from build123d import *

# Parameters (mm, degrees)
F1_DEPTH = 12
F2_W     = 13
F2_H     = 5.9
F3_DEPTH = 6
F4_W     = 13
F4_H     = 2.9
F5_DEPTH = 2
F6_W     = 2
F6_H     = 2.9
F7_DEPTH = 2


with BuildPart() as f1:
    # F0 (on Top) → F1 (new body)
    with BuildSketch(Plane.XY):
        Polygon((0, 3), (0, 0), (45, 0), (45, -5), (0, -5), (0, -13), (50, -13), (50, 3), align=None)
    extrude(amount=F1_DEPTH)

    # F2 (on face) → F3 (cut)
    with BuildSketch(Plane.XZ.offset(13)):
        with Locations((8.5, 6)):
            Rectangle(F2_W, F2_H)
    extrude(amount=-F3_DEPTH, mode=Mode.SUBTRACT)

    # F4 (on face) → F5 (cut, through all)
    with BuildSketch(Plane.XZ.offset(7)):
        with Locations((8.5, 6)):
            Rectangle(F4_W, F4_H)
    extrude(amount=-F5_DEPTH, mode=Mode.SUBTRACT)

    # F6 (on face) → F7 (cut, through all)
    with BuildSketch(Plane(origin=(0, 0, 0), x_dir=(0, -1, 0), z_dir=(-1, 0, 0))):
        with Locations((6, 6)):
            Rectangle(F6_W, F6_H)
    extrude(amount=-F7_DEPTH, mode=Mode.SUBTRACT)


solid = f1.part
CAD build for the part. Positions are in the model's coordinates, mm. A direction names the side the tool comes from. Give positions to 0.01 mm unless a question says otherwise; leave off trailing zeros. Order: outer loops, then holes, each group sorted by start corner. A loop starts at its lowest first (then second) coordinate and runs counter-clockwise, first axis right, second up. Notation, with made-up numbers: (85.25, 46) - (102.25, 46) arc R25 cw to (102.25, 71) - close; hole circle Ø2 at (-35.5, 11). An arc over 180 degrees is marked (long way). Write each question's results on one line, items separated by ' | '.
1. Saw through at A-A on y = -9.75. List the corners of the cut face in (x, z), and give its area (3 significant figures).
Calculated:
outline: (0, 0) - (50, 0) - (50, 12) - (0, 12) - close; hole (2, 3.05) - (15, 3.05) - (15, 8.95) - (2, 8.95) - close | area: 523 mm2
2. Pull direction Y, two halves, no side cores. Call faces 1 (the face through (1, -7, 6)), 2 (the face through (8, -7, 8)), 3 (the face through (2, -10, 6)): released by +Y, released by -Y, zero draft, split by the parting line, or undercut.
Calculated:
face 1: undercut | face 2: released by -Y | face 3: zero draft
3. Probe L1, parallel to Y at x = 33, z = 4; L2, parallel to Z at x = 6, y = -5.75; L3, parallel to Z at x = 11.5, y = -8.75. List the from-to ranges inside material, lowest first. Write a range as from..to.
Calculated:
L1: y = -13..-5, 0..3 | L2: z = 0..4.55, 7.45..12 | L3: z = 0..3.05, 8.95..12
4. Pin check, flat tip, straight feed: pin 1 (0.7 mm diameter, centred on x = 8.5, z = 8, fed in from -Y). Stop position of the tip, or through.
Calculated:
pin 1: stops at y = -7
5. Saw through at D-D on z = 2.25. List the corners of the cut face in (x, y), and give its area (3 significant figures).
Calculated:
outline: (0, -13) - (50, -13) - (50, 3) - (0, 3) - (0, 0) - (45, 0) - (45, -5) - (0, -5) - close | area: 575 mm2
6. 3-axis set-ups, long thin cutter, end or side, ignore diameter. For faces 4 (the face through (25, -7, 0)), 5 (the face through (45, -2, 6)), 6 (the face through (8, -10, 3.05)): which of +Z, -Z, +X, -X, +Y, -Y reach the whole face in a straight line?
Calculated:
face 4: -Z, +X, -X, +Y, -Y | face 5: +Z, -Z, -X | face 6: -Y
7. Saw through at C-C on z = 5.25. List the corners of the cut face in (x, y), and give its area (3 significant figures).
Calculated:
outline: (0, -13) - (2, -13) - (2, -7) - (0, -7) - close; (0, 0) - (45, 0) - (45, -5) - (15, -5) - (15, -13) - (50, -13) - (50, 3) - (0, 3) - close | area: 467 mm2
8. Saw through at B-B on x = 22. List the corners of the cut face in (y, z).
Calculated:
outline: (-13, 0) - (-5, 0) - (-5, 12) - (-13, 12) - close; (0, 0) - (3, 0) - (3, 12) - (0, 12) - close
